```python
from build123d import *

# Parameters (mm, degrees)
SKETCH1_R                  = 16.383
SKETCH1_R_2                = 14.986
BOSS_EXTRUDE1_DEPTH        = 3.4925
BOSS_EXTRUDE1_DEPTH_BACK   = 3.4925
SKETCH1_R_3                = 21.0058
SKETCH1_R_4                = 19.6088
BOSS_EXTRUDE1_2_DEPTH      = 3.4925
BOSS_EXTRUDE1_2_DEPTH_BACK = 3.4925
SKETCH1_3_R                = 19.6088
SKETCH1_3_R_2              = 16.383
BOSS_EXTRUDE2_DEPTH        = 3.1115
BOSS_EXTRUDE2_DEPTH_BACK   = 3.1115


with BuildPart() as part:
    # Sketch1 → Boss-Extrude1 (new body, two sides)
    with BuildSketch(Plane(origin=(0, 0, 0), x_dir=(1, 0, 0), z_dir=(0, 1, 0))) as boss_extrude1_sk:
        Circle(SKETCH1_R)
        Circle(SKETCH1_R_2, mode=Mode.SUBTRACT)
    extrude(amount=BOSS_EXTRUDE1_DEPTH)
    extrude(boss_extrude1_sk.sketch, amount=-BOSS_EXTRUDE1_DEPTH_BACK)



with BuildPart() as body_2:
    # Sketch1 → Boss-Extrude1 2 (new body, two sides)
    with BuildSketch(Plane(origin=(0, 0, 0), x_dir=(1, 0, 0), z_dir=(0, 1, 0))) as boss_extrude1_2_sk:
        Circle(SKETCH1_R_3)
        Circle(SKETCH1_R_4, mode=Mode.SUBTRACT)
    extrude(amount=BOSS_EXTRUDE1_2_DEPTH)
    extrude(boss_extrude1_2_sk.sketch, amount=-BOSS_EXTRUDE1_2_DEPTH_BACK)


with BuildPart() as part_1:
    add(part.part)

    add(body_2.part)  # Boss-Extrude2 merges body 2
    # Sketch1_3 → Boss-Extrude2 (add, two sides)
    with BuildSketch(Plane(origin=(0, 0, 0), x_dir=(1, 0, 0), z_dir=(0, 1, 0))) as boss_extrude2_sk:
        Circle(SKETCH1_3_R)
        Circle(SKETCH1_3_R_2, mode=Mode.SUBTRACT)
    extrude(amount=BOSS_EXTRUDE2_DEPTH)
    extrude(boss_extrude2_sk.sketch, amount=-BOSS_EXTRUDE2_DEPTH_BACK)


solid = part_1.part
```
Geometry: final body of the model. Coordinates: model frame, mm. A direction names the side the tool comes from. Coordinates: 2 decimals unless noted, no trailing zeros. Order: outer loops, then holes, each group sorted by start corner. A loop starts at its lowest first (then second) coordinate and runs counter-clockwise, first axis right, second up. Notation, with made-up numbers: (64, 26) - (103, 26) arc R34 cw to (103, 60) - close; hole circle Ø9 at (65, 53.25). An arc over 180 degrees is marked (long way). Return JSON: item names as keys, results as strings. Group by question number.
1. Set-up query: faces 4 (the face through (-6, -3.492, 19)), 5 (the face through (-12, -3.112, 12)), 6 (the face through (18.7, 3.3, -5.9)). Return all of +Z, -Z, +X, -X, +Y, -Y with unobstructed straight access to the full face (end or side cutting, diameter ignored); none if empty.
2. Cut plane C-C (y = 0). Output: boundary loops of the cut face in (x, z), plus the area to 3 significant figures.
3. Pin query (flat end, axial travel): pin 1 (1 mm diameter, centred on x = -11, y = -1.5, fed in from +Z); pin 2 (1.5 mm diameter, centred on y = -2.5, z = -16.5, fed in from -X). Return the tip coordinate at first contact, or that it passes through.
4. Pull-direction query (Z, two-part tool) for faces 1 (the face through (14.5, -3.492, 4.8)), 2 (the face through (20.036, 0.049, -6.31)), 3 (the face through (-12, 3.112, 12)); classes: pulls with the +Z half, pulls with the -Z half, needs draft (parallel to the pull), parting line crosses it, or undercut.
5. Cut plane A-A (z = 0). Output: boundary loops of the cut face in (x, y), plus the area to 3 significant figures.
6. Cut plane B-B (x = 0). Output: boundary loops of the cut face in (y, z), plus the area to 3 significant figures.
7. Material intervals for line 1 along X through (y, z) = (-3.4, 0); line 2 along Z through (x, y) = (0, 0.5), sorted ascending. Write a range as [from, to].
8. Cut plane D-D (x = -17). Output: boundary loops of the cut face in (y, z).
Resolved:
{
 "1": {"face 4": "+Z, -Z, +X, -X, -Y", "face 5": "-Y", "face 6": "+Y"},
 "2": {"outline": "circle Ø42.01 at (0, 0); hole circle Ø29.97 at (0, 0)", "area": "681 mm²"},
 "3": {"pin 1": "stops at z = 18.19", "pin 2": "stops at x = -13.9"},
 "4": {"face 1": "needs draft", "face 2": "parting line crosses it", "face 3": "undercut"},
 "5": {"outline": "(-21.01, -3.49) - (-19.61, -3.49) - (-19.61, -3.11) - (-16.38, -3.11) - (-16.38, -3.49) - (-14.99, -3.49) - (-14.99, 3.49) - (-16.38, 3.49) - (-16.38, 3.11) - (-19.61, 3.11) - (-19.61, 3.49) - (-21.01, 3.49) - close; (14.99, -3.49) - (16.38, -3.49) - (16.38, -3.11) - (19.61, -3.11) - (19.61, -3.49) - (21.01, -3.49) - (21.01, 3.49) - (19.61, 3.49) - (19.61, 3.11) - (16.38, 3.11) - (16.38, 3.49) - (14.99, 3.49) - close", "area": "79.2 mm²"},
 "6": {"outline": "(-3.49, -21.01) - (3.49, -21.01) - (3.49, -19.61) - (3.11, -19.61) - (3.11, -16.38) - (3.49, -16.38) - (3.49, -14.99) - (-3.49, -14.99) - (-3.49, -16.38) - (-3.11, -16.38) - (-3.11, -19.61) - (-3.49, -19.61) - close; (-3.49, 14.99) - (3.49, 14.99) - (3.49, 16.38) - (3.11, 16.38) - (3.11, 19.61) - (3.49, 19.61) - (3.49, 21.01) - (-3.49, 21.01) - (-3.49, 19.61) - (-3.11, 19.61) - (-3.11, 16.38) - (-3.49, 16.38) - close", "area": "79.2 mm²"},
 "7": {"line 1": "x = [-21.01, -19.61], [-16.38, -14.99], [14.99, 16.38], [19.61, 21.01]", "line 2": "z = [-21.01, -14.99], [14.99, 21.01]"},
 "8": {"outline": "(-3.49, -12.34) - (3.49, -12.34) - (3.49, -9.77) - (3.11, -9.77) - (3.11, 9.77) - (3.49, 9.77) - (3.49, 12.34) - (-3.49, 12.34) - (-3.49, 9.77) - (-3.11, 9.77) - (-3.11, -9.77) - (-3.49, -9.77) - close"}
}
